from build123d import *

# Parameters (mm, degrees)
SKETCH_W                           = 7.62
SKETCH_H                           = 10
PAD_DEPTH                          = 1.25
SKETCH001_W                        = 2.04
SKETCH001_H                        = 1.8
POCKET_DEPTH                       = 26.519708
SKETCH001_LINEARPATTERN_2_W        = 2.04
SKETCH001_LINEARPATTERN_2_H        = 1.8
POCKET_LINEARPATTERN_2_DEPTH       = 26.519708
SKETCH001_LINEARPATTERN_3_W        = 2.04
SKETCH001_LINEARPATTERN_3_H        = 1.8
POCKET_LINEARPATTERN_3_DEPTH       = 26.519708
SKETCH002_W                        = 2.04
SKETCH002_H                        = 3.38
POCKET001_DEPTH                    = 1.05
SKETCH002_LINEARPATTERN001_2_W     = 2.04
SKETCH002_LINEARPATTERN001_2_H     = 3.38
POCKET001_LINEARPATTERN001_2_DEPTH = 1.05
SKETCH002_LINEARPATTERN001_3_W     = 2.04
SKETCH002_LINEARPATTERN001_3_H     = 3.38
POCKET001_LINEARPATTERN001_3_DEPTH = 1.05
SKETCH003_W                        = 1.54
SKETCH003_H                        = 0.85
POCKET002_DEPTH                    = 4.9
SKETCH003_LINEARPATTERN002_2_W     = 1.54
SKETCH003_LINEARPATTERN002_2_H     = 0.85
POCKET002_LINEARPATTERN002_2_DEPTH = 4.9
SKETCH003_LINEARPATTERN002_3_W     = 1.54
SKETCH003_LINEARPATTERN002_3_H     = 0.85
POCKET002_LINEARPATTERN002_3_DEPTH = 4.9
SKETCH005_W                        = 0.2
SKETCH005_H                        = 2
POCKET003_DEPTH                    = 26.519708


with BuildPart() as part:
    # Sketch → Pad (new body)
    with BuildSketch(Plane.XY):
        Rectangle(SKETCH_W, SKETCH_H)
    extrude(amount=PAD_DEPTH)

    # Sketch001 → Pocket (cut, through all)
    with BuildSketch(Plane.XY):
        with Locations((-2.54, -4.1)):
            Rectangle(SKETCH001_W, SKETCH001_H)
    pocket = extrude(amount=POCKET_DEPTH, mode=Mode.SUBTRACT)

    # Sketch001 LinearPattern 2 → Pocket LinearPattern 2 (cut, through all)
    with BuildSketch(Plane(origin=(2.54, 0, 0), x_dir=(1, 0, 0), z_dir=(0, 0, 1))):
        with Locations((-2.54, -4.1)):
            Rectangle(SKETCH001_LINEARPATTERN_2_W, SKETCH001_LINEARPATTERN_2_H)
    pocket_linearpattern_2 = extrude(amount=POCKET_LINEARPATTERN_2_DEPTH, mode=Mode.SUBTRACT)

    # Sketch001 LinearPattern 3 → Pocket LinearPattern 3 (cut, through all)
    with BuildSketch(Plane(origin=(5.08, 0, 0), x_dir=(1, 0, 0), z_dir=(0, 0, 1))):
        with Locations((-2.54, -4.1)):
            Rectangle(SKETCH001_LINEARPATTERN_3_W, SKETCH001_LINEARPATTERN_3_H)
    pocket_linearpattern_3 = extrude(amount=POCKET_LINEARPATTERN_3_DEPTH, mode=Mode.SUBTRACT)

    # Mirrored: Pocket, Pocket LinearPattern 2, Pocket LinearPattern 3 across Sketch001 H_Axis
    add(pocket.mirror(Plane.ZX), mode=Mode.SUBTRACT)
    add(pocket_linearpattern_2.mirror(Plane.ZX), mode=Mode.SUBTRACT)
    add(pocket_linearpattern_3.mirror(Plane.ZX), mode=Mode.SUBTRACT)

    # Sketch002 → Pocket001 (cut)
    with BuildSketch(Plane.XY.offset(1.25)):
        with Locations((-2.54, -3.31)):
            Rectangle(SKETCH002_W, SKETCH002_H)
    pocket001 = extrude(amount=-POCKET001_DEPTH, mode=Mode.SUBTRACT)

    # Sketch002 LinearPattern001 2 → Pocket001 LinearPattern001 2 (cut)
    with BuildSketch(Plane(origin=(2.54, 0, 1.25), x_dir=(1, 0, 0), z_dir=(0, 0, 1))):
        with Locations((-2.54, -3.31)):
            Rectangle(SKETCH002_LINEARPATTERN001_2_W, SKETCH002_LINEARPATTERN001_2_H)
    pocket001_linearpattern001_2 = extrude(amount=-POCKET001_LINEARPATTERN001_2_DEPTH, mode=Mode.SUBTRACT)

    # Sketch002 LinearPattern001 3 → Pocket001 LinearPattern001 3 (cut)
    with BuildSketch(Plane(origin=(5.08, 0, 1.25), x_dir=(1, 0, 0), z_dir=(0, 0, 1))):
        with Locations((-2.54, -3.31)):
            Rectangle(SKETCH002_LINEARPATTERN001_3_W, SKETCH002_LINEARPATTERN001_3_H)
    pocket001_linearpattern001_3 = extrude(amount=-POCKET001_LINEARPATTERN001_3_DEPTH, mode=Mode.SUBTRACT)

    # Mirrored001: Pocket001, Pocket001 LinearPattern001 2, Pocket001 LinearPattern001 3 across Sketch002 H_Axis
    add(pocket001.mirror(Plane(origin=(0, 0, 1.25), x_dir=(0, 0, 1), z_dir=(0, 1, 0))), mode=Mode.SUBTRACT)
    add(pocket001_linearpattern001_2.mirror(Plane(origin=(0, 0, 1.25), x_dir=(0, 0, 1), z_dir=(0, 1, 0))), mode=Mode.SUBTRACT)
    add(pocket001_linearpattern001_3.mirror(Plane(origin=(0, 0, 1.25), x_dir=(0, 0, 1), z_dir=(0, 1, 0))), mode=Mode.SUBTRACT)

    # Sketch003 → Pocket002 (cut)
    with BuildSketch(Plane.XZ.offset(5)):
        with Locations((-2.54, 0.625)):
            Rectangle(SKETCH003_W, SKETCH003_H)
    pocket002 = extrude(amount=-POCKET002_DEPTH, mode=Mode.SUBTRACT)

    # Sketch003 LinearPattern002 2 → Pocket002 LinearPattern002 2 (cut)
    with BuildSketch(Plane(origin=(2.54, -5, 0), x_dir=(1, 0, 0), z_dir=(0, -1, 0))):
        with Locations((-2.54, 0.625)):
            Rectangle(SKETCH003_LINEARPATTERN002_2_W, SKETCH003_LINEARPATTERN002_2_H)
    pocket002_linearpattern002_2 = extrude(amount=-POCKET002_LINEARPATTERN002_2_DEPTH, mode=Mode.SUBTRACT)

    # Sketch003 LinearPattern002 3 → Pocket002 LinearPattern002 3 (cut)
    with BuildSketch(Plane(origin=(5.08, -5, 0), x_dir=(1, 0, 0), z_dir=(0, -1, 0))):
        with Locations((-2.54, 0.625)):
            Rectangle(SKETCH003_LINEARPATTERN002_3_W, SKETCH003_LINEARPATTERN002_3_H)
    pocket002_linearpattern002_3 = extrude(amount=-POCKET002_LINEARPATTERN002_3_DEPTH, mode=Mode.SUBTRACT)

    # Mirrored002: Pocket002, Pocket002 LinearPattern002 2, Pocket002 LinearPattern002 3 across XZ
    add(pocket002.mirror(Plane.XZ), mode=Mode.SUBTRACT)
    add(pocket002_linearpattern002_2.mirror(Plane.XZ), mode=Mode.SUBTRACT)
    add(pocket002_linearpattern002_3.mirror(Plane.XZ), mode=Mode.SUBTRACT)

    # Sketch005 → Pocket003 (cut, through all)
    with BuildSketch(Plane.XY):
        with Locations((-3.71, 0)):
            Rectangle(SKETCH005_W, SKETCH005_H)
    pocket003 = extrude(amount=POCKET003_DEPTH, mode=Mode.SUBTRACT)

    # Mirrored003: Pocket003 across Sketch005 V_Axis
    add(pocket003.mirror(Plane(origin=(0, 0, 0), x_dir=(0, 0, 1), z_dir=(1, 0, 0))), mode=Mode.SUBTRACT)


with BuildPart() as part_1:
    # Body placement: moved
    add(part.part.moved(Location((0, 0, 0.05))))


solid = part_1.part
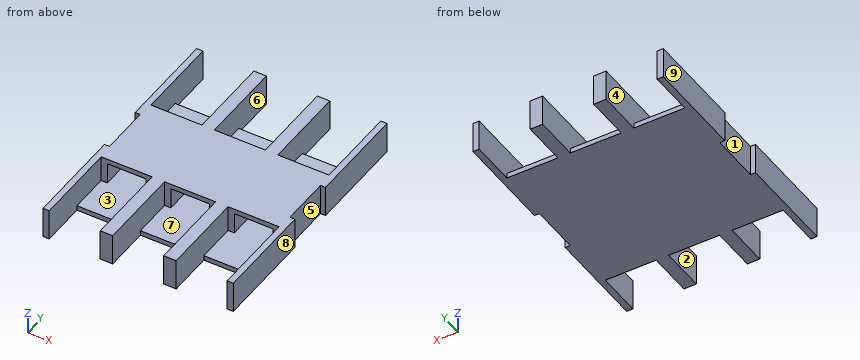
For this review, take the finished solid that the model builds, in its own axes (mm). Face numbers are marked on the shaded views. A direction names the side the tool comes from. Coordinates: 2 decimals unless noted, no trailing zeros. Write each loop counter-clockwise with the first axis right and the second up, starting at its lowest first coordinate (ties: lowest second). Pieces come first, ordered by that corner, then holes. Notation, with made-up numbers: (7.5, 11) -> (44.5, 11) arc R5 ccw to (44.5, 16) -> close; hole circle Ø11 at (28, 89.25). An arc over 180 degrees is marked (long way). Write each question's results on one line, items separated by ' | '. Start each with the question number.
1) Consider section A-A (y = -4.5). Write out the cut boundary in (x, z).
2) Consider section B-B (y = 1.25). Write out the cut boundary in (x, z).
3) Consider section C-C (x = -2.5). Write out the cut boundary in (y, z).
4) Wall thickness on L1, parallel to X at y = -2.75, z = 1; L2, parallel to X at y = -0.5, z = 0.85; L3, parallel to Z at x = 3, y = 1: over which ranges is each line inside the solid? List them lowest first. Write a range as [from, to].
5) Insertion check: pin 1 (0.7 mm diameter, centred on x = 0, z = 1, fed in from +Y). The pin has a flat end and moves straight along its axis. Give the tip position at first contact, or say it passes through.
6) For the marked faces 1, 2, 3, 4 and 5, list the 3-axis set-ups (+Z, -Z, +X, -X, +Y, -Y) from which the entire face can be reached by the end or side of a thin tool; tool diameter is ignored.
7) The part is to be moulded in two halves that separate along X. For the marked faces 6, 7, 8 and 9, say which applies: +X half, -X half, draft (parallel to the pull), parting line (faces both ways), or undercut.
Geometry says:
1) outline: (-3.81, 0.05) -> (-3.56, 0.05) -> (-3.56, 1.3) -> (-3.81, 1.3) -> close; (-1.52, 0.05) -> (-1.02, 0.05) -> (-1.02, 1.3) -> (-1.52, 1.3) -> close; (1.02, 0.05) -> (1.52, 0.05) -> (1.52, 1.3) -> (1.02, 1.3) -> close; (3.56, 0.05) -> (3.81, 0.05) -> (3.81, 1.3) -> (3.56, 1.3) -> close
2) outline: (-3.81, 0.05) -> (3.81, 0.05) -> (3.81, 1.3) -> (-3.81, 1.3) -> close; hole (-3.31, 0.25) -> (-1.77, 0.25) -> (-1.77, 1.1) -> (-3.31, 1.1) -> close; hole (-0.77, 0.25) -> (0.77, 0.25) -> (0.77, 1.1) -> (-0.77, 1.1) -> close; hole (1.77, 0.25) -> (3.31, 0.25) -> (3.31, 1.1) -> (1.77, 1.1) -> close
3) outline: (-3.2, 0.05) -> (3.2, 0.05) -> (3.2, 0.25) -> (0.1, 0.25) -> (0.1, 1.1) -> (1.62, 1.1) -> (1.62, 1.3) -> (-1.62, 1.3) -> (-1.62, 1.1) -> (-0.1, 1.1) -> (-0.1, 0.25) -> (-3.2, 0.25) -> close
4) L1: [-3.81, -3.56], [-1.52, -1.02], [1.02, 1.52], [3.56, 3.81] | L2: [-3.61, -3.31], [-1.77, -0.77], [0.77, 1.77], [3.31, 3.61] | L3: [0.05, 0.25], [1.1, 1.3]
5) pin 1: y = 1.62
6) face 1: +Z, -Z, -X | face 2: +Z, -Y | face 3: -Y | face 4: +Z, +Y | face 5: +Z, -Z, +X
7) face 6: undercut | face 7: undercut | face 8: +X half | face 9: -X half
